Geometry: final body of the model. Coordinates: model frame, mm. Face numbers are marked on the shaded views. A direction names the side the tool comes from. Give positions to 0.01 mm unless a question says otherwise; leave off trailing zeros. Order: outer loops, then holes, each group sorted by start corner. A loop starts at its lowest first (then second) coordinate and runs counter-clockwise, first axis right, second up. Notation, with made-up numbers: M 36,51.5 L 68,51.5 A32 cw 68,85.5 Z; hole C 19,-31.5 d5. An arc over 180 degrees is marked long. One line per item, written item: value. Start each with the question number.
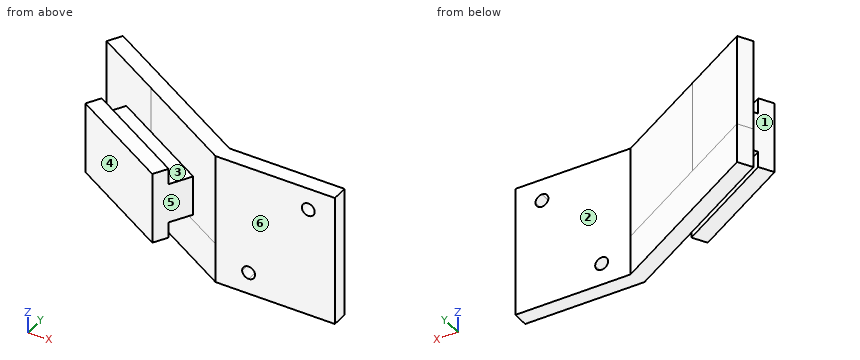
```python
from build123d import *

# Parameters (mm, degrees)
SKETCH1_W           = 50
SKETCH1_H           = 23
BOSS_EXTRUDE1_DEPTH = 20
CUT_EXTRUDE3_DEPTH  = 30
CUT_EXTRUDE4_DEPTH  = 30
SKETCH9_W           = 23
SKETCH9_H           = 4
BOSS_EXTRUDE2_DEPTH = 20
BOSS_EXTRUDE3_DEPTH = 10
SKETCH22_W          = 33
SKETCH22_H          = 4
BOSS_EXTRUDE4_DEPTH = 5
CUT_EXTRUDE7_DEPTH  = 5
SKETCH26_W          = 30
SKETCH26_H          = 10
BOSS_EXTRUDE5_DEPTH = 10
SKETCH28_W          = 30
SKETCH28_H          = 18
BOSS_EXTRUDE6_DEPTH = 4


with BuildPart() as part:
    # Sketch1 → Boss-Extrude1 (new body)
    with BuildSketch(Plane(origin=(0, 0, 0), x_dir=(1, 0, 0), z_dir=(0, 1, 0))):
        Rectangle(SKETCH1_W, SKETCH1_H)
    extrude(amount=BOSS_EXTRUDE1_DEPTH)

    # Sketch2 → Cut-Extrude3 (cut)
    with BuildSketch(Plane.XY.offset(11.5)):
        Polygon((0, 0), (-25, 14.43375673), (-25, 0), align=None)
        Polygon((1.07179677, 4), (25, 4), (25, 20), (-25, 20), (-25, 19.052558883), align=None)
    extrude(amount=-CUT_EXTRUDE3_DEPTH, mode=Mode.SUBTRACT)

    # Sketch4 → Cut-Extrude4 (cut)
    with BuildSketch(Plane.XY.offset(11.5)):
        Polygon((-25, 14.43375673), (-23, 17.897858345), (-25, 19.052558883), align=None)
    extrude(amount=-CUT_EXTRUDE4_DEPTH, mode=Mode.SUBTRACT)

    # Sketch9 → Boss-Extrude2 (add)
    with BuildSketch(Plane(origin=(-25, 14.43375673, 0), x_dir=(0, 0, 1), z_dir=(-0.8660254037844407, 0.4999999999999965, 0))):
        with Locations((0, 2)):
            Rectangle(SKETCH9_W, SKETCH9_H)
    extrude(amount=BOSS_EXTRUDE2_DEPTH)

    # Sketch11 → Boss-Extrude3 (add)
    with BuildSketch(Plane(origin=(0, 0, -11.5), x_dir=(-1, 0, 0), z_dir=(0, 0, -1))):
        Polygon((-25, 4), (-1.07179677, 4), (40.320508076, 27.897858345), (42.320508076, 24.43375673), (0, 0), (-25, 0), align=None)
    extrude(amount=BOSS_EXTRUDE3_DEPTH)

    # Sketch22 → Boss-Extrude4 (add)
    with BuildSketch(Plane(origin=(25, 0, 0), x_dir=(0, 0, -1), z_dir=(1, 0, 0))):
        with Locations((5, 2)):
            Rectangle(SKETCH22_W, SKETCH22_H)
    extrude(amount=BOSS_EXTRUDE4_DEPTH)

    # Sketch23 → Cut-Extrude7 (cut)
    with BuildSketch(Plane.XZ):
        with BuildLine():
            ThreePointArc((23.322235494, 7.62), (22.176722509, 4.854487014), (24.942235494, 6))
            Line((24.942235494, 6), (23.322235494, 6))
            Line((23.322235494, 6), (23.322235494, 7.62))
        make_face()
        with BuildLine():
            Line((23.322235494, 6), (24.942235494, 6))
            ThreePointArc((24.942235494, 6), (24.46774848, 7.145512986), (23.322235494, 7.62))
            Line((23.322235494, 7.62), (23.322235494, 6))
        make_face()
        with BuildLine():
            ThreePointArc((6.702235494, -16), (7.176722509, -17.145512986), (8.322235494, -17.62))
            Line((8.322235494, -17.62), (8.322235494, -16))
            Line((8.322235494, -16), (6.702235494, -16))
        make_face()
        with BuildLine():
            Line((8.322235494, -16), (8.322235494, -17.62))
            ThreePointArc((8.322235494, -17.62), (9.46774848, -17.145512986), (9.942235494, -16))
            ThreePointArc((9.942235494, -16), (8.322235494, -14.38), (6.702235494, -16))
            Line((6.702235494, -16), (8.322235494, -16))
        make_face()
    extrude(amount=-CUT_EXTRUDE7_DEPTH, mode=Mode.SUBTRACT)

    # Sketch26 → Boss-Extrude5 (add)
    with BuildSketch(Plane(origin=(0, 0, 0), x_dir=(0.8660254037844417, -0.4999999999999946, 0), z_dir=(-0.4999999999999946, -0.8660254037844417, 0))):
        with Locations((-25, -5)):
            Rectangle(SKETCH26_W, SKETCH26_H)
    extrude(amount=BOSS_EXTRUDE5_DEPTH)

    # Sketch28 → Boss-Extrude6 (add)
    with BuildSketch(Plane(origin=(-5, -8.660254038, 0), x_dir=(0.8660254037844417, -0.4999999999999946, 0), z_dir=(-0.4999999999999946, -0.8660254037844417, 0))):
        with Locations((-25, -5)):
            Rectangle(SKETCH28_W, SKETCH28_H)
    extrude(amount=-BOSS_EXTRUDE6_DEPTH)


solid = part.part
```
Q1. Contact query for flat-ended pins moving along their axis: pin 1 (10 mm diameter, centred on x = -29, y = 14, fed in from +Z); pin 2 (5.5 mm diameter, centred on x = -31.5, y = 7, fed in from +Z); pin 3 (1 mm diameter, centred on y = 20.5, z = -10, fed in from +X); pin 4 (5 mm diameter, centred on x = -17, z = -8.5, fed in from -Y). Output: stop coordinate, or through.
Q2. Section query A-A on z = -13. Return loops of the section in (x, y).
Q3. Ray query, line 1 along Y through (x, z) = (24.5, -13.5); line 2 along Y through (x, z) = (-22, -11); line 3 along X through (y, z) = (3.1, 6). Return the intervals inside material, ascending. Write a range as [from, to].
Q4. Section query D-D on x = -15. Return loops of the section in (y, z).
Q5. Section query B-B on y = 1.5. Return loops of the section in (x, z).
Q6. Set-up query: the marked faces 1, 2 and 3. Return all of +Z, -Z, +X, -X, +Y, -Y with unobstructed straight access to the full face (end or side cutting, diameter ignored); none if empty.
Q7. Mould query, pull axis X, two halves, no side actions, for the marked faces 4, 5 and 6. Classes: +X half, -X half, draft (parallel to the pull), parting line (faces both ways), or undercut.
Q8. Section query C-C on z = -2. Return loops of the section in (x, y), and give its area (3 significant figures).
Results below:
1. pin 1: z = 11.5
1. pin 2: z = 4
1. pin 3: x = -26.64
1. pin 4: y = -3.18
2. outline: M -42.32,24.43 L 0,0 L 30,0 L 30,4 L 1.07,4 L -40.32,27.9 Z; M -39.64,11.34 L -13.66,-3.66 L -11.66,-0.2 L -37.64,14.8 Z
3. line 1: [0, 4]
3. line 2: [1.15, 5.77], [12.7, 17.32]
3. line 3: [-5.37, 21.7], [24.94, 30]
4. outline: M -2.89,-14 L 1.73,-14 L 1.73,-10 L 8.66,-10 L 8.66,-21.5 L 13.28,-21.5 L 13.28,11.5 L 8.66,11.5 L 8.66,0 L 1.73,0 L 1.73,4 L -2.89,4 Z
5. outline: M -22.6,-14 L -14.6,-14 L -14.6,-10 L -10.68,-10 L -10.68,0 L -14.6,0 L -14.6,4 L -22.6,4 Z; M -2.6,-21.5 L 30,-21.5 L 30,11.5 L -2.6,11.5 Z; hole C 8.32,-16 d3.24; hole C 23.32,6 d3.24
6. face 1: +Z, -Z, -X
6. face 2: +Z, -Z, +X, +Y
6. face 3: +Z
7. face 4: -X half
7. face 5: undercut
7. face 6: draft
8. outline: M -42.32,24.43 L -34.64,20 L -39.64,11.34 L -13.66,-3.66 L -8.66,5 L 0,0 L 30,0 L 30,4 L 1.07,4 L -40.32,27.9 Z
8. area: 611 mm2
